```python
from build123d import *

# Parameters (mm, degrees)
SKETCH1_R           = 20
BOSS_EXTRUDE1_DEPTH = 30
SKETCH2_R           = 1.5
CUT_EXTRUDE1_DEPTH  = 18.5
CUT_EXTRUDE2_DEPTH  = 42.231056426
BOSS_EXTRUDE2_DEPTH = 40
SKETCH5_W           = 26.45751311
SKETCH5_H           = 5
CUT_EXTRUDE3_DEPTH  = 79.74007874


with BuildPart() as part:
    # Sketch1 → Boss-Extrude1 (new body)
    with BuildSketch(Plane(origin=(0, 0, 0), x_dir=(1, 0, 0), z_dir=(0, 1, 0))):
        with Locations(Location((0, 0, 0), (0, 0, 270))):
            Circle(SKETCH1_R)
        with BuildLine():
            Line((-2.452677109, 1.5), (2.452677109, 1.5))
            ThreePointArc((2.452677109, 1.5), (0, -2.875), (-2.452677109, 1.5))
        make_face(mode=Mode.SUBTRACT)
    extrude(amount=BOSS_EXTRUDE1_DEPTH)

    # Sketch2 → Cut-Extrude1 (cut)
    with BuildSketch(Plane(origin=(0, 0, -20), x_dir=(-1, 0, 0), z_dir=(0, 0, -1))):
        with Locations((0, 15)):
            Circle(SKETCH2_R)
    extrude(amount=-CUT_EXTRUDE1_DEPTH, mode=Mode.SUBTRACT)

    # Sketch3 → Cut-Extrude2 (cut, through all)
    with BuildSketch(Plane(origin=(0, 30, 0), x_dir=(1, 0, 0), z_dir=(0, 1, 0))):
        with BuildLine():
            ThreePointArc((-13.228756555, -15), (0, -20), (13.228756555, -15))
            Line((13.228756555, -15), (-13.228756555, -15))
        make_face()
        with BuildLine():
            Line((-13.228756555, 15), (13.228756555, 15))
            ThreePointArc((13.228756555, 15), (0, 20), (-13.228756555, 15))
        make_face()
    extrude(amount=-CUT_EXTRUDE2_DEPTH, mode=Mode.SUBTRACT)

    # Sketch4 → Boss-Extrude2 (add)
    with BuildSketch(Plane(origin=(0, 30, 0), x_dir=(1, 0, 0), z_dir=(0, 1, 0))):
        with BuildLine():
            Line((-13.228756555, -15), (13.228756555, -15))
            ThreePointArc((13.228756555, -15), (20, 0), (13.228756555, 15))
            Line((13.228756555, 15), (-13.228756555, 15))
            ThreePointArc((-13.228756555, 15), (-20, 0), (-13.228756555, -15))
        make_face()
        with BuildLine():
            Line((-2.452677109, 1.5), (2.452677109, 1.5))
            ThreePointArc((2.452677109, 1.5), (0, -2.875), (-2.452677109, 1.5))
        make_face(mode=Mode.SUBTRACT)
    extrude(amount=BOSS_EXTRUDE2_DEPTH)

    # Sketch5 → Cut-Extrude3 (cut, through all)
    with BuildSketch(Plane.XY.offset(15)):
        with Locations((0, 67.5)):
            Rectangle(SKETCH5_W, SKETCH5_H)
        with BuildLine():
            Line((13.228756555, 65), (-13.228756555, 65))
            Line((-13.228756555, 65), (-13.228756555, 62.928932188))
            ThreePointArc((-13.228756555, 62.928932188), (0, 55), (13.228756555, 62.928932188))
            Line((13.228756555, 62.928932188), (13.228756555, 65))
        make_face()
        with BuildLine():
            Line((14.142135624, 75), (-14.142135624, 75))
            ThreePointArc((-14.142135624, 75), (-15, 70), (-14.142135624, 65))
            Line((-14.142135624, 65), (-13.228756555, 65))
            Line((-13.228756555, 65), (-13.228756555, 70))
            Line((-13.228756555, 70), (13.228756555, 70))
            Line((13.228756555, 70), (13.228756555, 65))
            Line((13.228756555, 65), (14.142135624, 65))
            ThreePointArc((14.142135624, 65), (14.783978395, 67.463470319), (15, 70))
            ThreePointArc((15, 70), (14.783978395, 72.536529681), (14.142135624, 75))
        make_face()
        with BuildLine():
            Line((20, 75), (14.142135624, 75))
            ThreePointArc((14.142135624, 75), (14.783978395, 72.536529681), (15, 70))
            ThreePointArc((15, 70), (14.783978395, 67.463470319), (14.142135624, 65))
            Line((14.142135624, 65), (20, 65))
            Line((20, 65), (20, 75))
        make_face()
        with BuildLine():
            ThreePointArc((13.228756555, 62.928932188), (13.72456794, 63.947212637), (14.142135624, 65))
            Line((14.142135624, 65), (13.228756555, 65))
            Line((13.228756555, 65), (13.228756555, 62.928932188))
        make_face()
        with BuildLine():
            Line((-14.142135624, 75), (-20, 75))
            Line((-20, 75), (-20, 65))
            Line((-20, 65), (-14.142135624, 65))
            ThreePointArc((-14.142135624, 65), (-15, 70), (-14.142135624, 75))
        make_face()
    extrude(amount=-CUT_EXTRUDE3_DEPTH, mode=Mode.SUBTRACT)


solid = part.part
```
Model file for the job. Use its own axes, mm. A direction names the side the tool comes from. Round coordinates to 2 decimals unless told otherwise and drop trailing zeros. Write each loop counter-clockwise with the first axis right and the second up, starting at its lowest first coordinate (ties: lowest second). Pieces come first, ordered by that corner, then holes. Notation, with made-up numbers: (16.5, -13) - (46.5, -13) arc R34 cw to (46.5, 17) - close; hole circle Ø4 at (39, 32.25). An arc over 180 degrees is marked (long way). One line per item, written item: value.
(1) Cut at D-D, the plane x = 15. Give the cut face in (y, z).
Values follow:
outline: (0, -13.23) - (65, -13.23) - (65, 13.23) - (0, 13.23) - close
(2) Cut at B-B, the plane x = 0. Give the cut face in (y, z) (3 decimals).
Values follow:
outline: (0, -15) - (13.5, -15) - (13.5, -1.5) - (0, -1.5) - close; (0, 2.875) - (55, 2.875) - (55, 15) - (0, 15) - close; (16.5, -15) - (55, -15) - (55, -1.5) - (16.5, -1.5) - close
(3) 3-axis set-ups, long thin cutter, end or side, ignore diameter. For faces 3 (the flat face through (-13.229, 64, 0)), 4 (the cylindrical face through (1.11, 16.01, -8.34)), 5 (the flat face through (-16, 65, 0)), 6 (the flat face through (0, 27, -1.5)): which of +Z, -Z, +X, -X, +Y, -Y reach the whole face in a straight line?
Values follow:
face 3: +Z, -Z, +Y
face 4: -Z
face 5: +Z, -Z, +X, -X, +Y
face 6: +Y, -Y
(4) Cut at A-A, the plane z = 0. Give the cut face in (x, y) (3 decimals).
Values follow:
outline: (-20, 0) - (-2.875, 0) - (-2.875, 55.278) arc R15 cw to (-13.229, 62.929) - (-13.229, 65) - (-20, 65) - close; (2.875, 0) - (20, 0) - (20, 65) - (14.142, 65) arc R15 cw to (2.875, 55.278) - close
(5) Drop flat-ended pins along their axis: P1, Ø3, axis at x = -2, z = -11.5, coming from the +Y side; P2, Ø1.8, axis at x = 0, y = 15, coming from the -Z side; P3, Ø6, axis at y = 18.5, z = -8, coming from the +X side. Give the stop position or say it passes through.
Values follow:
P1: stops at y = 55.41
P2: stops at z = 2.73
P3: stops at x = 19.36
(6) Cut at C-C, the plane y = 15. Give the cut face in (x, z) (3 decimals), plus the area to 3 significant figures.
Values follow:
outline: (-13.229, -15) - (-1.5, -15) - (-1.5, -1.5) - (-2.453, -1.5) arc R2.875 cw (long way) to (2.453, -1.5) - (1.5, -1.5) - (1.5, -15) - (13.229, -15) arc R20 ccw to (13.229, 15) - (-13.229, 15) arc R20 ccw to start
area: 1,010 mm²
(7) Two-plate mould, pull along X, no slides. Class faces 1 (the flat face through (16, 65, 0)), 2 (the cylindrical face through (0.085, 27.255, 2.874)): pulls with the +X half, pulls with the -X half, needs draft (parallel to the pull), parting line crosses it, or undercut.
Values follow:
face 1: needs draft
face 2: undercut
(8) Wall check: probe 1 along Z at (x, y) = (0, 36) (3 decimals); probe 2 along X at (y, z) = (28.5, 0) (3 decimals); probe 3 along Z at (x, y) = (15, 33.5). Give the ranges that are in metal, low to high.
Values follow:
probe 1: z = -15 to -1.5, 2.875 to 15
probe 2: x = -20 to -2.875, 2.875 to 20
probe 3: z = -13.23 to 13.23
